Could you check a few things on this model? Use its own coordinates, in mm. Give positions to 0.01 mm unless a question says otherwise; leave off trailing zeros. Write each loop counter-clockwise with the first axis right and the second up, starting at its lowest first coordinate (ties: lowest second). Pieces come first, ordered by that corner, then holes. Notation, with made-up numbers: (-24.5, 30) -> (23.5, 30) arc R22 cw to (23.5, 40) -> close; hole circle Ø3 at (-23, 21.5). An arc over 180 degrees is marked (long way). One line per question, with ' | ' between items.
from build123d import *

# Parameters (mm, degrees)
F0_W     = 34.29
F0_H     = 369.824
F0_W_2   = 221.488
F0_H_2   = 30.48
F1_DEPTH = 3
F2_W     = 212.566798
F2_H     = 309.88
F2_W_2   = 19.780282
F2_W_3   = 22.356551
F2_W_4   = 86.36
F2_H_2   = 5.08
F2_R     = 2.5
F2_R_2   = 3.81
F2_W_5   = 57.019912
F3_DEPTH = 25.4
F5_DEPTH = 25.4


with BuildPart() as f1:
    # F0 (on Front) → F1 (new body)
    with BuildSketch(Plane.XZ):
        with Locations((-263.71608, 0.16686)):
            Rectangle(F0_W, F0_H)
        with BuildLine():
            Line((-246.57108, 191.42886), (-246.57108, 185.07886))
            Line((-246.57108, 185.07886), (-246.57108, -184.74514))
            Line((-246.57108, -184.74514), (-246.57108, -191.09514))
            ThreePointArc((-246.57108, -191.09514), (-240.991464, -204.565524), (-227.52108, -210.14514))
            Line((-227.52108, -210.14514), (-221.17108, -210.14514))
            Line((-221.17108, -210.14514), (0.31692, -210.14514))
            Line((0.31692, -210.14514), (0.31692, 210.47886))
            Line((0.31692, 210.47886), (-202.12108, 210.47886))
            Line((-202.12108, 210.47886), (-221.17108, 210.47886))
            Line((-221.17108, 210.47886), (-227.52108, 210.47886))
            ThreePointArc((-227.52108, 210.47886), (-240.991464, 204.899244), (-246.57108, 191.42886))
        make_face()
        Polygon((-221.17108, 240.95886), (-221.17108, 210.47886), (-202.12108, 210.47886), (0.31692, 210.47886), (0.31692, 240.95886), align=None)
        with Locations((-110.42708, -225.38514)):
            Rectangle(F0_W_2, F0_H_2)
    extrude(amount=F1_DEPTH)

    # F2 (on Front) → F3 (cut)
    with BuildSketch(Plane.XZ):
        with Locations((-126.063681, 41.31486)):
            Rectangle(F2_W, F2_H)
        with Locations((-9.890141, 41.31486)):
            Rectangle(F2_W_2, F2_H)
        with Locations((11.178275, 41.31486)):
            Rectangle(F2_W_3, F2_H)
        Polygon((-261.367738, -166.503845), (-271.527738, -153.803845), (-271.527738, -160.153845), (-261.367738, -172.853845), align=None)
        Polygon((-271.527738, -134.753845), (-271.527738, -141.103845), (-261.367738, -153.803845), (-261.367738, -147.453845), align=None)
        Polygon((-271.527738, -122.053845), (-261.367738, -134.753845), (-261.367738, -128.403845), (-271.527738, -115.703845), align=None)
        Polygon((-271.527738, -103.003845), (-261.367738, -115.703845), (-261.367738, -109.353845), (-271.527738, -96.653845), align=None)
        Polygon((-271.527738, -83.953845), (-261.367738, -96.653845), (-261.367738, -90.303845), (-271.527738, -77.603845), align=None)
        Polygon((-271.527738, -64.903845), (-261.367738, -77.603845), (-261.367738, -71.253845), (-271.527738, -58.553845), align=None)
        Polygon((-271.527738, -45.853845), (-261.367738, -58.553845), (-261.367738, -52.203845), (-271.527738, -39.503845), align=None)
        Polygon((-271.527738, -26.803845), (-261.367738, -39.503845), (-261.367738, -33.153845), (-271.527738, -20.453845), align=None)
        with Locations((-150.390271, -228.668471)):
            Rectangle(F2_W_4, F2_H_2)
        with Locations((-150.390271, -219.778471)):
            Rectangle(F2_W_4, F2_H_2)
        with Locations((-48.790271, -219.778471)):
            Rectangle(F2_W_4, F2_H_2)
        with Locations((-48.790271, -228.668471)):
            Rectangle(F2_W_4, F2_H_2)
        with Locations((-206.757738, -223.780845)):
            Circle(F2_R)
        with Locations((-81.97908, 203.87486)):
            Circle(F2_R_2)
        with Locations((-238.69708, 40.658346)):
            Circle(F2_R_2)
        with Locations((0, -119.97514)):
            Circle(F2_R_2)
        with Locations((-2.669124, 203.87486)):
            Rectangle(F2_W_5, F2_H_2)
    extrude(amount=F3_DEPTH, mode=Mode.SUBTRACT)

    # F4 (on Front) → F5 (cut)
    with BuildSketch(Plane.XZ):
        Polygon((-224.760328, -128.296434), (-231.110328, -128.296434), (-154.910328, -194.336434), (-148.560328, -194.336434), align=None)
        Polygon((-205.710328, -128.296434), (-212.060328, -128.296434), (-154.910328, -177.826434), (-148.560328, -177.826434), align=None)
        Polygon((-224.760328, -145.913435), (-231.110328, -145.913435), (-175.237637, -194.336434), (-168.887637, -194.336434), align=None)
        Polygon((-224.760328, -161.858131), (-231.110328, -161.858131), (-193.635364, -194.336434), (-187.285364, -194.336434), align=None)
        Polygon((-224.760328, -177.031307), (-231.110328, -177.031307), (-211.142873, -194.336434), (-204.792873, -194.336434), align=None)
        Polygon((-154.910328, -163.62169), (-148.560328, -163.62169), (-189.320239, -128.296434), (-195.670239, -128.296434), align=None)
        Polygon((-154.910328, -148.76998), (-148.560328, -148.76998), (-172.183651, -128.296434), (-178.533651, -128.296434), align=None)
    extrude(amount=F5_DEPTH, mode=Mode.SUBTRACT)


solid = f1.part
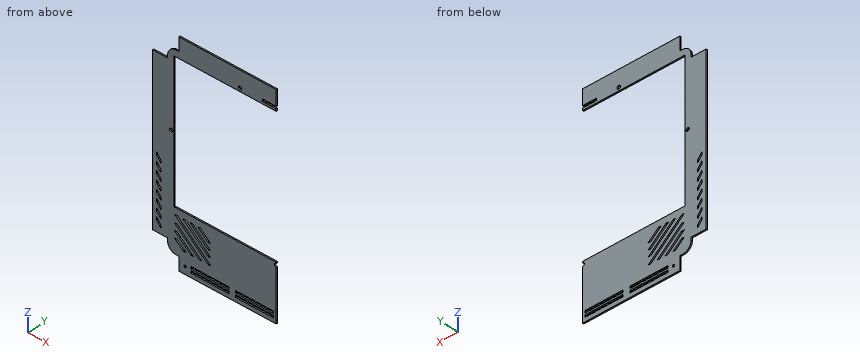
Q1. Imagine slicing it at B-B on y = -0.75. Count the separate pieces of the cut face and the enclosed holes in it, and give its area (3 significant figures).
Answer below:
separate pieces: 1 | enclosed holes: 22 | area: 53,500 mm^2
Q2. Will these pins go through, and if not, where does the flat tip stop? pin 1 (7 mm diameter, centred on x = 0, z = -119.98, fed in from +Y); pin 2 (1.5 mm diameter, centred on y = -2, z = -220, fed in from -X); pin 3 (1.5 mm diameter, centred on y = -2, z = -187, fed in from -X).
Answer below:
pin 1: passes through | pin 2: stops at x = -221.17 | pin 3: stops at x = -246.57
Q3. If I drill on line 1 along Z through (x, y) = (-57.5, -1.8); line 2 along Z through (x, y) = (-17, -1.8); line 3 along Z through (x, y) = (-227, -1.5), over which ranges is the centre line in solid material (lowest first)?
Answer below:
line 1: z = -240.63 to -231.21, -226.13 to -222.32, -217.24 to -113.63, 196.25 to 240.96 | line 2: z = -240.63 to -231.21, -226.13 to -222.32, -217.24 to -113.63, 196.25 to 201.33, 206.41 to 240.96 | line 3: z = -210.15 to -180.59, -177.03 to -165.42, -161.86 to -149.48, -145.91 to -131.86, -128.3 to -113.63, 196.25 to 210.48
Q4. Imagine slicing it at A-A on z = 102. Please give me the cut outline in (x, y), and give its area (3 significant figures).
Answer below:
outline: (-280.86, -3) -> (-232.35, -3) -> (-232.35, 0) -> (-280.86, 0) -> close | area: 146 mm^2
